Geometry: final body of the model. Coordinates: model frame, mm. A direction names the side the tool comes from. Round coordinates to 2 decimals unless told otherwise and drop trailing zeros. Loops run counter-clockwise (first coordinate to the right, second up) from the corner with the lowest first, then second, coordinate; pieces in that order, holes last. Notation, with made-up numbers: (-24, 21) - (16, 21) arc R15 ccw to (16, 25) - close; hole circle Ø6 at (-33, -15). An arc over 180 degrees is marked (long way). Use CSV: the item, a comma, the result in double quotes.
from build123d import *

# Parameters (mm, degrees)
SKETCH1_W            = 32.5
SKETCH1_H            = 3
SKETCH1_W_2          = 6
SKETCH1_H_2          = 7
M3_CLEARANCE_HOLE1_D = 3.4
CUT_EXTRUDE1_DEPTH   = 12.5
CIRPATTERN1_COUNT    = 14


with BuildPart() as part:
    # Sketch1 → Revolve1 (revolve)
    with BuildSketch(Plane(origin=(0, 0, 0), x_dir=(1, 0, 0), z_dir=(0, 1, 0))):
        Polygon((45, 1.5), (45, -1.5), (45, -10), (50, -10), (50, 10), (45, 10), align=None)
        with Locations((28.75, 0)):
            Rectangle(SKETCH1_W, SKETCH1_H)
        with Locations((9.5, 0)):
            Rectangle(SKETCH1_W_2, SKETCH1_H_2)
    revolve(axis=Axis((0, 0, 77.742212382), (0, 0, -1)))

    # M3 Clearance Hole1 (through all)
    with Locations(Plane.XY.offset(3.5)):
        with Locations((-4.75, 8.227241336), (4.75, 8.227241336), (9.5, 0), (4.75, -8.227241336), (-4.75, -8.227241336), (-9.5, 0)):
            Hole(M3_CLEARANCE_HOLE1_D / 2)

    # Sketch5 → Cut-Extrude1 (cut, through all)
    with BuildSketch(Plane.XY.offset(1.5)):
        with BuildLine():
            ThreePointArc((14.488887394, 3.882285677), (14.871672921, 1.957892883), (15, 0))
            ThreePointArc((15, 0), (32.542393706, 12.411508104), (26.676923077, 33.084615385))
            ThreePointArc((26.676923077, 33.084615385), (27.759031054, 15.488385465), (14.488887394, 3.882285677))
        make_face()
    cut_extrude1 = extrude(amount=-CUT_EXTRUDE1_DEPTH, mode=Mode.SUBTRACT)

    # CirPattern1: Cut-Extrude1 ×14 about axis
    cirpattern1_axis = Axis((0, 0, 0), (0, 0, 1))
    for i in range(1, CIRPATTERN1_COUNT):
        add(cut_extrude1.rotate(cirpattern1_axis, i * 360 / CIRPATTERN1_COUNT), mode=Mode.SUBTRACT)


solid = part.part
Item 1: Material intervals for line 1 (Y direction, x = -6, z = -2); line 2 (X direction, y = 31.5, z = -1); line 3 (X direction, y = -40, z = 0.75), sorted ascending.
Final values:
line 1,"y = -49.64 to -44.6, -10.97 to -9.38, -7.08 to -2.5, 2.5 to 7.08, 9.38 to 10.97, 44.6 to 49.64"
line 2,"x = -38.83 to -10.45, -1.24 to 5.12, 11.52 to 17.21, 22.13 to 27.49, 28.41 to 38.83"
line 3,"x = -30 to -13.58, -11.46 to -3.06, 4.2 to 30"
Item 2: Section A-A on z = 8.5. Return the cut outline in (x, y), plus the area to 3 significant figures.
Final values:
outline,"circle Ø100 at (0, 0); hole circle Ø90 at (0, 0)"
area,"1,490 mm²"
Item 3: Pin query (flat end, axial travel): P1, Ø4, axis at y = 36.5, z = 3, coming from the +X side; P2, Ø4, axis at x = 34, z = 6.5, coming from the +Y side; P3, Ø2, axis at x = 9.5, y = 0, coming from the -Z side; P4, Ø4, axis at y = -14, z = -6.5, coming from the +X side. Return the tip coordinate at first contact, or that it passes through.
Final values:
P1,"stops at x = 36.19"
P2,"stops at y = 38.42"
P3,"passes through"
P4,"stops at x = 48.54"
Item 4: Reachability of faces 4 (the cylindrical face through (-10.82, 10.39, 0.02)), 5 (the cylindrical face through (20.765, 39.923, -5.69)), 6 (the flat face through (41, -19, 10)) from +Z, -Z, +X, -X, +Y, -Y: full face, straight path, thin tool, end or side. Return the list, or none.
Final values:
face 4,"+Z, -Z"
face 5,"-Z"
face 6,"+Z, +X, -X, +Y, -Y"
Item 5: Mould query, pull axis Y, two halves, no side actions, for faces 1 (the cylindrical face through (-29.69, 17.807, 0.021)), 2 (the cylindrical face through (47.69, -15.02, -0.14)), 3 (the flat face through (-41, -19, -10)). Classes: released by +Y, released by -Y, zero draft, split by the parting line, or undercut.
Final values:
face 1,"undercut"
face 2,"split by the parting line"
face 3,"zero draft"
Item 6: Section B-B on y = 20.5. Give the number of separate pieces and of enclosed holes in the cut face, plus the area to 3 significant figures.
Final values:
separate pieces,"7"
enclosed holes,"0"
area,"371 mm²"
